Check sheet for the drawn part. Datum: minimum x, y, z corner. Units: mm. Coordinates: 2 decimals unless noted, no trailing zeros. Order: outer loops, then holes, each group sorted by start corner. A loop starts at its lowest first (then second) coordinate and runs counter-clockwise, first axis right, second up.
Q1. Cross-section at D-D, the plane z = 45.5. Record the boundary of the cut face in (x, y).
Q2. Cross-section at B-B, the plane x = 96. Record the boundary of the cut face in (y, z).
Q3. Draft check along Z on the marked faces 1, 2 and 3. Enter one of: pulls with the +Z half, pulls with the -Z half, needs draft (parallel to the pull), parting line crosses it, or undercut.
Q4. Depth check by flat-ended pin: P1, Ø7, axis at x = 19.51, z = 45.5, coming from the -Y side; P2, Ø6, axis at y = 10.5, z = 91, coming from the -X side; P3, Ø1, axis at x = 35.5, y = 12.5, coming from the -Z side; P4, Ø1, axis at x = 116.5, y = 5.5, coming from the +Z side. Enter the tip coordinate at first touch or a pass-through.
Q5. Thickness scan on line 1 (X direction, y = 9.75, z = 116.5); line 2 (Y direction, x = 84, z = 135); line 3 (X direction, y = 8.75, z = 115). Record the ranges inside material, lowest first.
Q6. Cross-section at C-C, the plane y = 5.5. Count the separate pieces of the cut face and the enclosed holes in it, and give its area (3 significant figures).
Q7. Cross-section at A-A, the plane z = 81. Record the boundary of the cut face in (x, y) (3 decimals), and give its area (3 significant figures).
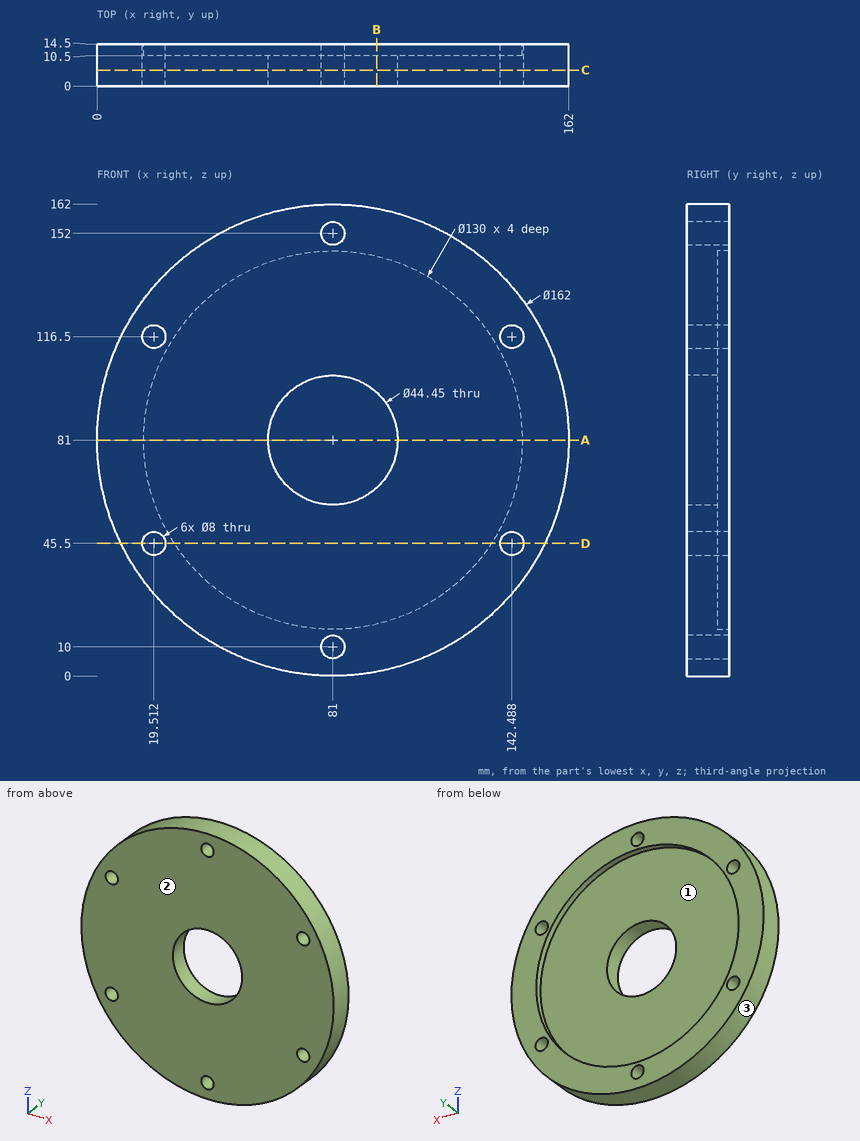
Check values:
1. outline: (8.19, 0) - (15.51, 0) - (15.51, 14.5) - (8.19, 14.5) - close; (23.51, 0) - (138.49, 0) - (138.49, 14.5) - (135.45, 14.5) - (135.45, 10.5) - (26.55, 10.5) - (26.55, 14.5) - (23.51, 14.5) - close; (146.49, 0) - (153.81, 0) - (153.81, 14.5) - (146.49, 14.5) - close
2. outline: (0, 1.4) - (14.5, 1.4) - (14.5, 17.75) - (10.5, 17.75) - (10.5, 64.6) - (0, 64.6) - close; (0, 97.4) - (10.5, 97.4) - (10.5, 144.25) - (14.5, 144.25) - (14.5, 160.6) - (0, 160.6) - close
3. face 1: undercut
3. face 2: needs draft
3. face 3: parting line crosses it
4. P1: passes through
4. P2: stops at x = 0.3
4. P3: stops at z = 13.65
4. P4: stops at z = 154.05
5. line 1: x = 8.19 to 15.51, 23.51 to 138.49, 146.49 to 153.81
5. line 2: y = 0 to 10.5
5. line 3: x = 7.48 to 15.8, 23.22 to 138.78, 146.2 to 154.52
6. separate pieces: 1
6. enclosed holes: 7
6. area: 18,800 mm2
7. outline: (0, 0) - (58.775, 0) - (58.775, 10.5) - (16, 10.5) - (16, 14.5) - (0, 14.5) - close; (103.225, 0) - (162, 0) - (162, 14.5) - (146, 14.5) - (146, 10.5) - (103.225, 10.5) - close
7. area: 1,360 mm2
